Autodesk Inventor part; units mm, degrees
ref_plane "YZ Plane" through (0, 0, 0) normal (1, 0, 0) x (0, 1, 0)
ref_plane "XZ Plane" through (0, 0, 0) normal (0, 1, 0) x (-1, 0, 0)
ref_plane "XY Plane" through (0, 0, 0) normal (0, 0, 1) x (1, 0, 0)
sketch "Sketch1" plane through (0, 0, 0) normal (0, 0, 1) x (1, 0, 0)
  line L0 (2519.2496, -500.1029) -> (2519.2496, -385.3529)
  line L1 (2554.2496, -380.3529) -> (2524.2496, -380.3529)
  line L2 (2554.2496, -380.3529) -> (2554.2496, -515.3529)
  line L3 (2467.7344, -543.3529) -> (2524.2496, -543.3529)
  line L4 (2554.2496, -515.3529) -> (2524.2496, -543.3529)
  line L5 (2514.9996, -504.3529) -> (2467.7344, -504.3529)
  line L6 (2467.7344, -543.3529) -> (2467.7344, -504.3529)
  line L7 (2521.7496, -380.3529) -> (2519.2496, -384.3529)
  arc A0 (2514.9996, -504.3529) -> (2519.2496, -500.1029) centre (2519.2496, -504.3529) ccw
  line L8 (2519.2496, -385.3529) -> (2524.2496, -380.3529)
  point P0 (0, 0)
  point P1 (2519.2496, -380.3529)
  dimension "d1" = 35
  dimension "d3" = 135
  dimension "d5" = 163
  dimension "d7" = 51.5152
  dimension "d9" = 39
  dimension "d11" = 56.5152
  dimension "d13" = 8.5
  dimension "d16" = 5
  dimension "d17" = 5
extrude "Extrusion1" add sketch "Sketch1" along normal blind 5
properties part number "ADSK-MH-10038" material "Steel, Mild"
Model file for the job. Use its own axes, mm. Give positions to 0.01 mm unless a question says otherwise; leave off trailing zeros. Loops run counter-clockwise (first coordinate to the right, second up) from the corner with the lowest first, then second, coordinate; pieces in that order, holes last. Notation, with made-up numbers: (22.25, -8.75) - (74.25, -8.75) arc R31 ccw to (74.25, 27.25) - close; hole circle Ø7 at (69.25, 60). An arc over 180 degrees is marked (long way). One line per item, written item: value. Start each with the question number.
1. Probe L1, parallel to X at y = -406, z = 4; L2, parallel to Y at x = 2479, z = 0.65; L3, parallel to X at y = -506, z = 4.75. List the from-to ranges inside material, lowest first. Write a range as from..to.
2. Pin check, flat tip, straight feed: pin 1 (1 mm diameter, centred on y = -490.5, z = 1.5, fed in from -X). Stop position of the tip, or through.
3. Pull direction X, two halves, no side cores. Call faces 1 (the flat face through (2492, -504.353, 2)), 2 (the flat face through (2519.25, -444, 2)), 3 (the cylindrical face through (2522.35, -507.26, 2.46)): pulls with the +X half, pulls with the -X half, needs draft (parallel to the pull), parting line crosses it, or undercut.
4. Slice it at B-B (x = 2540). List the corners of the cut face in (y, z).
5. Slice it at C-C (y = -446.5). List the corners of the cut face in (x, z), plus the area to 3 significant figures.
6. Slice it at A-A (z = 3.8). List the corners of the cut face in (x, y).
Solution:
1. L1: x = 2519.25..2554.25
1. L2: y = -543.35..-504.35
1. L3: x = 2467.73..2515.33, 2523.17..2554.25
2. pin 1: stops at x = 2519.25
3. face 1: needs draft
3. face 2: pulls with the -X half
3. face 3: undercut
4. outline: (-528.65, 0) - (-380.35, 0) - (-380.35, 5) - (-528.65, 5) - close
5. outline: (2519.25, 0) - (2554.25, 0) - (2554.25, 5) - (2519.25, 5) - close
5. area: 175 mm^2
6. outline: (2467.73, -543.35) - (2524.25, -543.35) - (2554.25, -515.35) - (2554.25, -380.35) - (2524.25, -380.35) - (2519.25, -385.35) - (2519.25, -500.1) arc R4.25 cw (long way) to (2515, -504.35) - (2467.73, -504.35) - close
